```python
from build123d import *

# Parameters (mm, degrees)
SKETCH1_W           = 62
SKETCH1_H           = 38
BOSS_EXTRUDE1_DEPTH = 26
SKETCH2_W           = 58
SKETCH2_H           = 35
CUT_EXTRUDE1_DEPTH  = 17
SKETCH4_W           = 45
SKETCH4_H           = 35
CUT_EXTRUDE3_DEPTH  = 7
SKETCH5_R           = 6.375
CUT_EXTRUDE4_DEPTH  = 9
SKETCH6_W           = 9.989337028
SKETCH6_H           = 25
CUT_EXTRUDE5_DEPTH  = 17
SKETCH7_R           = 3.375
CUT_EXTRUDE6_DEPTH  = 7
SKETCH8_W           = 9
SKETCH8_H           = 4
CUT_EXTRUDE7_DEPTH  = 7
FILLET1_R           = 2.5


with BuildPart() as part:
    # Sketch1 → Boss-Extrude1 (new body)
    with BuildSketch(Plane.XY):
        with Locations((31, 19)):
            Rectangle(SKETCH1_W, SKETCH1_H)
    extrude(amount=BOSS_EXTRUDE1_DEPTH)

    # Sketch2 → Cut-Extrude1 (cut)
    with BuildSketch(Plane.XY.offset(26)):
        with Locations((31, 19)):
            Rectangle(SKETCH2_W, SKETCH2_H)
    extrude(amount=-CUT_EXTRUDE1_DEPTH, mode=Mode.SUBTRACT)

    # Sketch4 → Cut-Extrude3 (cut)
    with BuildSketch(Plane.XY.offset(9)):
        with Locations((31, 19)):
            Rectangle(SKETCH4_W, SKETCH4_H)
    extrude(amount=-CUT_EXTRUDE3_DEPTH, mode=Mode.SUBTRACT)

    # Sketch5 → Cut-Extrude4 (cut)
    with BuildSketch(Plane(origin=(0, 0, 0), x_dir=(-1, 0, 0), z_dir=(0, 0, -1))):
        with Locations((-54, 19)):
            Circle(SKETCH5_R)
        with Locations((-8, 19)):
            Circle(SKETCH5_R)
    extrude(amount=-CUT_EXTRUDE4_DEPTH, mode=Mode.SUBTRACT)

    # Sketch6 → Cut-Extrude5 (cut)
    with BuildSketch(Plane(origin=(62, 0, 0), x_dir=(0, 0, -1), z_dir=(1, 0, 0))):
        with Locations((-15.005331486, 19)):
            Rectangle(SKETCH6_W, SKETCH6_H)
    extrude(amount=-CUT_EXTRUDE5_DEPTH, mode=Mode.SUBTRACT)

    # Sketch7 → Cut-Extrude6 (cut)
    with BuildSketch(Plane.ZY):
        with Locations((18, 19)):
            Circle(SKETCH7_R)
    extrude(amount=-CUT_EXTRUDE6_DEPTH, mode=Mode.SUBTRACT)

    # Sketch8 → Cut-Extrude7 (cut)
    with BuildSketch(Plane.XZ):
        with Locations((30.5, 17)):
            Rectangle(SKETCH8_W, SKETCH8_H)
    extrude(amount=-CUT_EXTRUDE7_DEPTH, mode=Mode.SUBTRACT)

    # Fillet1
    fillet1_edges = [part.edges().sort_by_distance(p)[0] for p in [
        (0, 38, 13),
        (62, 38, 13),
        (62, 0, 13),
        (0, 0, 13),
    ]]
    fillet(fillet1_edges, radius=FILLET1_R)


solid = part.part
```
Input: part model. Units: mm. Frame: model coordinates. A direction names the side the tool comes from. Give positions to 0.01 mm unless a question says otherwise; leave off trailing zeros. Order: outer loops, then holes, each group sorted by start corner. A loop starts at its lowest first (then second) coordinate and runs counter-clockwise, first axis right, second up. Notation, with made-up numbers: M 20.25,26 L 66.25,26 A16 ccw 66.25,31 Z; hole C 51,24.5 d10. An arc over 180 degrees is marked long. One line per question, with ' | ' between items.
1) Access query for faces 4 (the face through (61, 31.5, 15)), 5 (the face through (30, 1, 15)), 6 (the face through (57, 8, 9)). Directions: +Z, -Z, +X, -X, +Y, -Y. A direction counts if a zero-diameter tool reaches every point of the face in a straight line with its end or side. Return the directions, or none.
Filled in:
face 4: +X | face 5: -Y | face 6: +Z
2) Section C-C on y = 19. Output: boundary loops of the cut face in (x, z) (3 decimals), and give its area (3 significant figures).
Filled in:
outline: M 0,0 L 1.625,0 L 1.625,9 L 2,9 L 2,14.625 L 0,14.625 Z; M 0,21.375 L 2,21.375 L 2,26 L 0,26 Z; M 14.375,0 L 47.625,0 L 47.625,2 L 14.375,2 Z; M 60,9 L 60.375,9 L 60.375,0 L 62,0 L 62,10.011 L 60,10.011 Z; M 60,20 L 62,20 L 62,26 L 60,26 Z | area: 130 mm2
3) Section B-B on z = 18. Output: boundary loops of the cut face in (x, y) (3 decimals).
Filled in:
outline: M 0,2.5 A2.5 ccw 2.5,0 L 26,0 L 26,1.5 L 2,1.5 L 2,15.625 L 0,15.625 Z; M 0,22.375 L 2,22.375 L 2,36.5 L 60,36.5 L 60,31.5 L 62,31.5 L 62,35.5 A2.5 ccw 59.5,38 L 2.5,38 A2.5 ccw 0,35.5 Z; M 35,0 L 59.5,0 A2.5 ccw 62,2.5 L 62,6.5 L 60,6.5 L 60,1.5 L 35,1.5 Z
4) Draft query along Z for faces 1 (the face through (2, 19, 14)), 2 (the face through (0.99, 19.15, 14.63)), 3 (the face through (31, 19, 0)). Return one class per face: pulls with the +Z half, pulls with the -Z half, needs draft (parallel to the pull), parting line crosses it, or undercut.
Filled in:
face 1: needs draft | face 2: undercut | face 3: pulls with the -Z half
5) Section A-A on x = 34. Output: boundary loops of the cut face in (y, z).
Filled in:
outline: M 0,0 L 38,0 L 38,26 L 36.5,26 L 36.5,2 L 1.5,2 L 1.5,15 L 0,15 Z; M 0,19 L 1.5,19 L 1.5,26 L 0,26 Z
6) Section D-D on z = 6.75. Output: boundary loops of the cut face in (x, y) (3 decimals).
Filled in:
outline: M 0,2.5 A2.5 ccw 2.5,0 L 59.5,0 A2.5 ccw 62,2.5 L 62,35.5 A2.5 ccw 59.5,38 L 2.5,38 A2.5 ccw 0,35.5 Z; hole M 8.5,1.5 L 53.5,1.5 L 53.5,12.645 A6.375 ccw long 53.5,25.355 L 53.5,36.5 L 8.5,36.5 L 8.5,25.355 A6.375 ccw long 8.5,12.645 Z
7) Ray query, L1, parallel to X at y = 4, z = 9.25; L2, parallel to X at y = 35, z = 5; L3, parallel to Y at x = 9, z = 24.25. Return the intervals inside material, ascending.
Filled in:
L1: x = 0 to 2, 60 to 62 | L2: x = 0 to 8.5, 53.5 to 62 | L3: y = 0 to 1.5, 36.5 to 38
8) Contact query for flat-ended pins moving along their axis: P1, Ø1.6, axis at y = 0.5, z = 18, coming from the -X side; P2, Ø6, axis at y = 19, z = 18, coming from the -X side; P3, Ø7.5, axis at x = 8, y = 19, coming from the +Z side; P4, Ø2, axis at x = 58, y = 29, coming from the +Z side. Output: stop coordinate, or through.
Filled in:
P1: stops at x = 0.31 | P2: stops at x = 60 | P3: passes through | P4: stops at z = 9
